Autodesk Inventor part; units mm, degrees
ref_plane "YZ Plane" through (0, 0, 0) normal (1, 0, 0) x (0, 1, 0)
ref_plane "XZ Plane" through (0, 0, 0) normal (0, 1, 0) x (-1, 0, 0)
ref_plane "XY Plane" through (0, 0, 0) normal (0, 0, 1) x (1, 0, 0)
sketch "Sketch1" plane through (0, 0, 0) normal (0, 1, 0) x (-1, 0, 0)
  line L0 (0, 0) -> (48, 0)
  line L1 (48, 0) -> (48, -18)
  line L2 (48, -18) -> (0, -18)
  line L3 (0, -18) -> (0, 0)
  dimension "d0" = 48
  dimension "d1" = 18
extrude "Extrusion1" add sketch "Sketch1" along normal blind 15
sketch "Sketch2" plane through (0, 15, 0) normal (0, 1, 0) x (1, 0, 0)
  line L0 (-48, 18) -> (-48, 0)
  line L1 (-48, 0) -> (-42.5, 0)
  line L2 (-48, 0) -> (0, 0)
  line L3 (-42.5, 0) -> (-42.5, 2)
  line L4 (-42.5, 2) -> (-29.5, 2)
  line L5 (-29.5, 2) -> (-29.5, 16)
  line L6 (-42.5, 2) -> (-42.5, 16)
  line L7 (-42.5, 16) -> (-29.5, 16)
  dimension "d4" = 5.5
  dimension "d5" = 2
  dimension "d6" = 13
  dimension "d7" = 14
extrude "Extrusion2" cut sketch "Sketch2" against normal blind 5
sketch "Sketch3" plane through (0, 0, 0) normal (1, 0, 0) x (0, 0, -1)
  line L0 (0, 0) -> (0, 15)
  line L1 (0, 15) -> (18, 15)
  line L2 (16, 15) -> (2, 15)
  line L3 (9, 15) -> (9, 11.5)
  line L4 (9, 11.5) -> (13.1, 11.5)
  line L5 (13.1, 11.5) -> (4.9, 11.5)
  line L6 (4.9, 11.5) -> (4.9, 8.25)
  line L7 (4.9, 8.25) -> (13.1, 8.25)
  line L8 (13.1, 8.25) -> (13.1, 11.5)
  line L9 (16, 10) -> (2, 10)
  line L10 (4.9, 10) -> (7.1782, 7.7218)
  line L11 (4.9, 10) -> (8.1218, 10) construction
  line L12 (13.1, 10) -> (10.403, 7.303)
  line L13 (13.1, 10) -> (16.9142, 10) construction
  point P0 (11.35, 8.25)
  point P1 (6.65, 8.25)
  dimension "d10" = 18
  dimension "d11" = 3.5
  dimension "d12" = 4.1
  dimension "d13" = 8.2
  dimension "d14" = 3.25
  dimension "d15" = 45
  dimension "d16" = 135
extrude "Extrusion3" cut sketch "Sketch3" against normal blind 5 contours L4 L8 L9 L6 L5 | L12 L7 L10 L9
properties part number "U2D2"
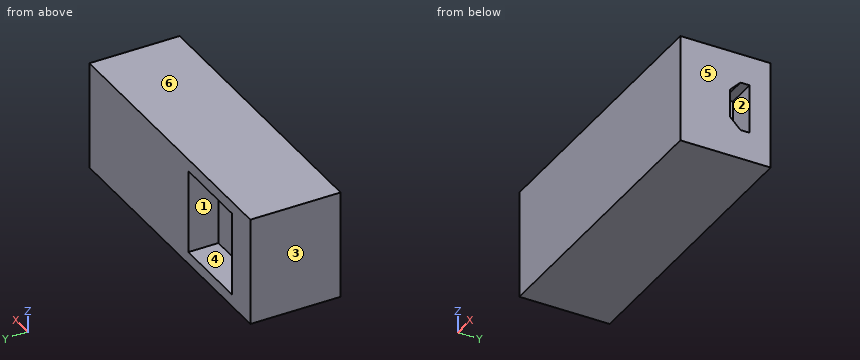
Build history of the part. All positions in model axes, mm. Face numbers are marked on the shaded views. A direction names the side the tool comes from. Give positions to 0.01 mm unless a question says otherwise; leave off trailing zeros. Loops run counter-clockwise (first coordinate to the right, second up) from the corner with the lowest first, then second, coordinate; pieces in that order, holes last.
Item 1: Slice it at B-B, the plane x = -4. List the corners of the cut face in (y, z), and give its area (3 significant figures).
Answers follow:
outline: (0, -18) - (15, -18) - (15, 0) - (0, 0) - close; hole (8.25, -11.35) - (10, -13.1) - (11.5, -13.1) - (11.5, -4.9) - (10, -4.9) - (8.25, -6.65) - close
area: 246 mm2
Item 2: Drill centre lines: line 1 (Z direction, x = -42, y = 13); line 2 (X direction, y = 14, z = -4.25); line 3 (X direction, y = 8.5, z = -8.75). Where is each one in solid material? Low to high.
Answers follow:
line 1: z = -18 to -16, -2 to 0
line 2: x = -48 to -42.5, -29.5 to 0
line 3: x = -48 to -5
Item 3: Which spindle directions (+Z, -Z, +X, -X, +Y, -Y) get a long thin tool onto all of the face, cutting with end or side? Do the marked faces 1, 2 and 3. Say none if no direction does.
Answers follow:
face 1: +Y
face 2: +X
face 3: +Z, -Z, -X, +Y, -Y
Item 4: Slice it at C-C, the plane z = -6. List the corners of the cut face in (x, y), and give its area (3 significant figures).
Answers follow:
outline: (-48, 0) - (0, 0) - (0, 8.9) - (-5, 8.9) - (-5, 11.5) - (0, 11.5) - (0, 15) - (-29.5, 15) - (-29.5, 10) - (-42.5, 10) - (-42.5, 15) - (-48, 15) - close
area: 642 mm2
Item 5: Slice it at D-D, the plane x = -37. List the corners of the cut face in (y, z), and give its area (3 significant figures).
Answers follow:
outline: (0, -18) - (15, -18) - (15, -16) - (10, -16) - (10, -2) - (15, -2) - (15, 0) - (0, 0) - close
area: 200 mm2
Item 6: Flat gauge pins, fed straight in: pin 1 (1 mm diameter, centred on y = 10.5, z = -10.5, fed in from +X); pin 2 (3 mm diameter, centred on x = -37.5, z = -7.5, fed in from +Y). Where does each tip first touch, or does it go through?
Answers follow:
pin 1: stops at x = -5
pin 2: stops at y = 10
Item 7: Pull direction Z, two halves, no side cores. Call the marked faces 4, 5 and 6: released by +Z, released by -Z, zero draft, split by the parting line, or undercut.
Answers follow:
face 4: undercut
face 5: zero draft
face 6: released by +Z
Item 8: Slice it at A-A, the plane y = 12.75. List the corners of the cut face in (x, z), and give its area (3 significant figures).
Answers follow:
outline: (-48, -18) - (0, -18) - (0, 0) - (-48, 0) - close; hole (-42.5, -16) - (-29.5, -16) - (-29.5, -2) - (-42.5, -2) - close
area: 682 mm2
